```python
from build123d import *

# Parameters (mm, degrees)
ESBO_O1_W                = 10
ESBO_O1_H                = 18
RESSALTO_EXTRUS_O1_DEPTH = 6
RESSALTO_EXTRUS_O2_DEPTH = 8
FILETE1_R                = 0.5
ESBO_O3_W                = 8
ESBO_O3_H                = 17
CORTE_EXTRUS_O1_DEPTH    = 13
RESSALTO_EXTRUS_O3_REACH = 12
ESBO_O4_R                = 1.25
ESBO_O5_R                = 0.75
CORTE_EXTRUS_O2_DEPTH    = 11
CORTE_EXTRUS_O3_REACH    = 20
ESBO_O6_R                = 0.75
RESSALTO_EXTRUS_O6_REACH = 19
ESBO_O7_W                = 14.6
ESBO_O7_H                = 8.7


with BuildPart() as part:
    # Esboço1 → Ressalto-extrusão1 (new body, symmetric)
    with BuildSketch(Plane(origin=(0, 0, 0), x_dir=(1, 0, 0), z_dir=(0, 1, 0))):
        Rectangle(ESBO_O1_W, ESBO_O1_H)
    extrude(amount=RESSALTO_EXTRUS_O1_DEPTH, both=True)

    # Esboço2 → Ressalto-extrusão2 (add)
    with BuildSketch(Plane(origin=(5, 0, 0), x_dir=(0, 0, -1), z_dir=(1, 0, 0))):
        with BuildLine():
            Line((3.5, 1.118033989), (3.5, -1.118033989))
            ThreePointArc((3.5, -1.118033989), (6, 0), (3.5, 1.118033989))
        make_face()
    extrude(amount=RESSALTO_EXTRUS_O2_DEPTH)

    # Filete1
    filete1_edges = [part.edges().sort_by_distance(p)[0] for p in [
        (0, -6, -9),
        (0, 6, -9),
    ]]
    fillet(filete1_edges, radius=FILETE1_R)

    # Esboço3 → Corte-extrusão1 (cut, through all)
    with BuildSketch(Plane(origin=(0, 6, 0), x_dir=(1, 0, 0), z_dir=(0, 1, 0))):
        with Locations((0, 0.5)):
            Rectangle(ESBO_O3_W, ESBO_O3_H)
    extrude(amount=-CORTE_EXTRUS_O1_DEPTH, mode=Mode.SUBTRACT)

    # Esboço4 → Ressalto-extrusão3 (add, up to next)
    with BuildSketch(Plane(origin=(5, 0, 0), x_dir=(0, 0, -1), z_dir=(1, 0, 0)), mode=Mode.PRIVATE) as ressalto_extrus_o3_sk1:
        with Locations((7.35, 4.35)):
            Circle(ESBO_O4_R)
    ressalto_extrus_o3_tool1 = extrude(ressalto_extrus_o3_sk1.sketch, amount=-RESSALTO_EXTRUS_O3_REACH, mode=Mode.PRIVATE) - part.part
    add(ressalto_extrus_o3_tool1.solids().sort_by_distance((5, 4.35, -7.35))[0])
    # Esboço4 → Ressalto-extrusão3 (add, up to next)
    with BuildSketch(Plane(origin=(5, 0, 0), x_dir=(0, 0, -1), z_dir=(1, 0, 0)), mode=Mode.PRIVATE) as ressalto_extrus_o3_sk2:
        with Locations((7.35, -4.35)):
            Circle(ESBO_O4_R)
    ressalto_extrus_o3_tool2 = extrude(ressalto_extrus_o3_sk2.sketch, amount=-RESSALTO_EXTRUS_O3_REACH, mode=Mode.PRIVATE) - part.part
    add(ressalto_extrus_o3_tool2.solids().sort_by_distance((5, -4.35, -7.35))[0])

    # Esboço5 → Corte-extrusão2 (cut, through all)
    with BuildSketch(Plane(origin=(5, 0, 0), x_dir=(0, 0, -1), z_dir=(1, 0, 0))):
        with Locations((7.35, 4.35)):
            Circle(ESBO_O5_R)
        with Locations((7.35, -4.35)):
            Circle(ESBO_O5_R)
    extrude(amount=-CORTE_EXTRUS_O2_DEPTH, mode=Mode.SUBTRACT)

    # Esboço6 → Corte-extrusão3 (cut, up to next)
    with BuildSketch(Plane.XY.offset(9), mode=Mode.PRIVATE) as corte_extrus_o3_sk1:
        Circle(ESBO_O6_R)
    corte_extrus_o3_tool1 = extrude(corte_extrus_o3_sk1.sketch, amount=-CORTE_EXTRUS_O3_REACH, mode=Mode.PRIVATE) & part.part
    add(corte_extrus_o3_tool1.solids().sort_by_distance((0, 0, 9))[0], mode=Mode.SUBTRACT)

    # Esboço7 → Ressalto-extrusão6 (add, up to next)
    with BuildSketch(Plane(origin=(-4, 0, 0), x_dir=(0, 0, -1), z_dir=(1, 0, 0)), mode=Mode.PRIVATE) as ressalto_extrus_o6_sk1:
        with Locations((-0.7, 0)):
            Rectangle(ESBO_O7_W, ESBO_O7_H)
    ressalto_extrus_o6_tool1 = extrude(ressalto_extrus_o6_sk1.sketch, amount=RESSALTO_EXTRUS_O6_REACH, mode=Mode.PRIVATE) - part.part
    add(ressalto_extrus_o6_tool1.solids().sort_by_distance((-4, 0, 0.7))[0])


solid = part.part
```
Geometry: final body of the model. Coordinates: model frame, mm. A direction names the side the tool comes from. Round coordinates to 2 decimals unless told otherwise and drop trailing zeros. Loops run counter-clockwise (first coordinate to the right, second up) from the corner with the lowest first, then second, coordinate; pieces in that order, holes last. Notation, with made-up numbers: (3.25, 8.25) -> (48.25, 8.25) arc R21 cw to (48.25, 42.25) -> close; hole circle Ø9 at (38, 2.5). An arc over 180 degrees is marked (long way). Use one line per item in the form item = value.
Item 1: Cut plane C-C on z = -4.5. Output: boundary loops of the cut face in (x, y).
Evaluation:
outline = (-5, -6) -> (-4, -6) -> (-4, -4.35) -> (4, -4.35) -> (4, -6) -> (5, -6) -> (5, -1.5) -> (13, -1.5) -> (13, 1.5) -> (5, 1.5) -> (5, 6) -> (4, 6) -> (4, 4.35) -> (-4, 4.35) -> (-4, 6) -> (-5, 6) -> close
Item 2: Cut plane D-D on x = 3.25. Output: boundary loops of the cut face in (y, z).
Evaluation:
outline = (-6, 8) -> (-4.35, 8) -> (-4.35, -6.1) arc R1.25 ccw (long way) to (-3.35, -6.6) -> (3.35, -6.6) arc R1.25 ccw (long way) to (4.35, -6.1) -> (4.35, 8) -> (6, 8) -> (6, 9) -> (-6, 9) -> close; hole circle Ø1.5 at (-4.35, -7.35); hole circle Ø1.5 at (4.35, -7.35)
Item 3: Contact query for flat-ended pins moving along their axis: pin 1 Ø2 at (x, y) = (1, 0.5) entering from -Z; pin 2 Ø5 at (y, z) = (-4, -7) entering from +X; pin 3 Ø2 at (x, z) = (2.5, -3.5) entering from -Y. Output: stop coordinate, or through.
Evaluation:
pin_1 = -6.6
pin_2 = 5
pin_3 = -4.35
Item 4: Draft query along Z for faces 4 (the flat face through (5, 0, 0)), 5 (the flat face through (1, 0, 9)), 6 (the cylindrical face through (0.056, -4.951, -8.446)). Return one class per face: released by +Z, released by -Z, zero draft, split by the parting line, or undercut.
Evaluation:
face_4 = zero draft
face_5 = released by +Z
face_6 = undercut
Item 5: Cut plane B-B on y = 2.25. Output: boundary loops of the cut face in (x, z), then the cut area to 3 significant figures.
Evaluation:
outline = (-5, -9) -> (-4, -9) -> (-4, -6.6) -> (4, -6.6) -> (4, -9) -> (5, -9) -> (5, 9) -> (-5, 9) -> close
area = 161 mm2
Item 6: Cut plane A-A on x = 0. Output: boundary loops of the cut face in (y, z).
Evaluation:
outline = (-6, 8) -> (-4.35, 8) -> (-4.35, -6.1) arc R1.25 ccw (long way) to (-3.35, -6.6) -> (3.35, -6.6) arc R1.25 ccw (long way) to (4.35, -6.1) -> (4.35, 8) -> (6, 8) -> (6, 9) -> (0.75, 9) -> (0.75, 8) -> (-0.75, 8) -> (-0.75, 9) -> (-6, 9) -> close; hole circle Ø1.5 at (-4.35, -7.35); hole circle Ø1.5 at (4.35, -7.35)
Item 7: Access query for faces 1 (the flat face through (-4, 4.5, -1.7)), 2 (the cylindrical face through (9, 0, -6)), 3 (the flat face through (0, 5, 8)). Directions: +Z, -Z, +X, -X, +Y, -Y. A direction counts if a zero-diameter tool reaches every point of the face in a straight line with its end or side. Return the directions, or none.
Evaluation:
face_1 = none
face_2 = +X
face_3 = +Y
Item 8: Material intervals for probe 1 along Y at (x, z) = (2.75, -7.35); probe 2 along X at (y, z) = (-4.75, 7); probe 3 along Y at (x, z) = (1, 7.25), sorted ascending.
Evaluation:
probe_1 = -5.6 to -5.1, -3.6 to -3.1, 3.1 to 3.6, 5.1 to 5.6
probe_2 = -5 to -4, 4 to 5
probe_3 = -4.35 to 4.35
